Input: part model. Units: mm. Frame: model coordinates. A direction names the side the tool comes from. Coordinates: 2 decimals unless noted, no trailing zeros. Order: outer loops, then holes, each group sorted by start corner. A loop starts at its lowest first (then second) coordinate and runs counter-clockwise, first axis right, second up. Notation, with made-up numbers: (-23.5, 26) -> (11.5, 26) arc R23 cw to (11.5, 38) -> close; hole circle Ø5 at (-1, 16). An arc over 180 degrees is marked (long way). Use one line per item in the form item = value. Start each with the question number.
1) Access query for faces 1 (the flat face through (15.49, 31.73, 524.63)), 2 (the flat face through (-66, 0, 593)). Directions: +Z, -Z, +X, -X, +Y, -Y. A direction counts if a zero-diameter tool reaches every point of the face in a straight line with its end or side. Return the directions, or none.
2) Pin query (flat end, axial travel): pin 1 (12 mm diameter, centred on x = -97.5, y = -110, fed in from +Z); pin 2 (13.5 mm diameter, centred on x = -142, z = 668.5, fed in from -Y); pin 3 (2 mm diameter, centred on y = -3.5, z = 733, fed in from -X). Return the tip coordinate at first contact, or that it passes through.
3) Section query A-A on y = -34. Count the separate pieces of the cut face and the enclosed holes in it, then the cut area to 3 significant figures.
4) Section query B-B on y = 77. Output: boundary loops of the cut face in (x, z).
5) Ray query, line 1 along Z through (x, y) = (-135, 13); line 2 along Y through (x, z) = (-300, 820.5); line 3 along X through (y, z) = (65, 487). Return the intervals inside material, ascending.
6) Section query C-C on z = 561.5. Output: boundary loops of the cut face in (x, y).
from build123d import *

# Parameters (mm, degrees)
F1_DEPTH = 152.4
F2_W     = 19.05
F2_H     = 152.4
F3_DEPTH = 19.05


with BuildPart() as f1:
    # F0 (on Front) → F1 (new body, symmetric)
    with BuildSketch(Plane.XZ):
        Polygon((-371.3216865451, 884.5013463886), (378.5296995641, 134.6499602793), (378.5296995641, 161.5907286425), (-357.8513023635, 897.9717305702), align=None)
    extrude(amount=F1_DEPTH, both=True)

    # F2 (on face) → F3 (cut)
    with BuildSketch(Plane(origin=(270.0602141033, 0, 270.0602141033), x_dir=(0.7071067812, 0, -0.7071067812), z_dir=(0.7071067812, 0, 0.7071067812))):
        with Locations((74.0240174423, -76.2)):
            Rectangle(F2_W, F2_H)
        with Locations((-33.9259825577, -76.2)):
            Rectangle(F2_W, F2_H)
        with Locations((-141.8759825577, -76.2)):
            Rectangle(F2_W, F2_H)
        with Locations((-249.8259825577, -76.2)):
            Rectangle(F2_W, F2_H)
        with Locations((-357.7759825577, -76.2)):
            Rectangle(F2_W, F2_H)
        with Locations((-465.7259825577, -76.2)):
            Rectangle(F2_W, F2_H)
        with Locations((-573.6759825577, -76.2)):
            Rectangle(F2_W, F2_H)
        with Locations((-681.6259825577, -76.2)):
            Rectangle(F2_W, F2_H)
        with Locations((-789.5759825577, -76.2)):
            Rectangle(F2_W, F2_H)
    extrude(amount=-F3_DEPTH, mode=Mode.SUBTRACT)


solid = f1.part
Answers below:
q1.face_1 = +Z, +X, +Y, -Y
q1.face_2 = -Y
q2.pin_1 = 643.62
q2.pin_2 = 0
q2.pin_3 = -218.49
q3.separate_pieces = 10
q3.enclosed_holes = 0
q3.area = 16,800 mm^2
q4.outline = (-371.32, 884.5) -> (378.53, 134.65) -> (378.53, 161.59) -> (-357.85, 897.97) -> close
q5.line_1 = 648.18 to 675.12
q5.line_2 = 0 to 152.4
q5.line_3 = 26.18 to 53.12
q6.outline = (-48.32, -152.4) -> (-21.38, -152.4) -> (-21.38, 152.4) -> (-48.32, 152.4) -> close
